Input: part model. Units: mm. Frame: model coordinates. A direction names the side the tool comes from. Coordinates: 2 decimals unless noted, no trailing zeros. Order: outer loops, then holes, each group sorted by start corner. A loop starts at its lowest first (then second) coordinate and runs counter-clockwise, first axis right, second up.
Autodesk Inventor part; units mm, degrees
ref_plane "YZ Plane" through (0, 0, 0) normal (1, 0, 0) x (0, 1, 0)
ref_plane "XZ Plane" through (0, 0, 0) normal (0, 1, 0) x (-1, 0, 0)
ref_plane "XY Plane" through (0, 0, 0) normal (0, 0, 1) x (1, 0, 0)
sketch "Boceto1" plane through (0, 0, 0) normal (0, 0, 1) x (1, 0, 0)
  line L0 (-19.271, 0) -> (-1.6402, 0)
  circle A0 centre (-16, 0) radius 2.75
  circle A1 centre (16, 0) radius 2.75
  line L1 (21, -7) -> (-21, -7)
  line L2 (-21, -7) -> (-21, 7)
  line L3 (-21, 7) -> (21, 7)
  line L4 (21, 7) -> (21, -7)
  line L5 (21, -7) -> (-21, 7) construction
  line L6 (-21, -7) -> (21, 7) construction
  point P0 (0, 0)
  point P1 (0, 0)
  dimension "d0" = 5.5
  dimension "d1" = 5.5
  dimension "d2" = 16
  dimension "d3" = 32
  dimension "d4" = 14
  dimension "d5" = 42
extrude "Extrusión1" add sketch "Boceto1" along normal blind 6
sketch "Boceto2" plane through (0, 0, 6) normal (0, 0, 1) x (1, 0, 0)
  point P0 (0, 0)
sketch "Boceto3" plane through (0, 0, 0) normal (0, 1, 0) x (-1, 0, 0)
  line L0 (-21, 0) -> (21, 0)
  line L1 (-8.586, 32.8) -> (-8.586, 0)
  line L2 (-8.586, 0) -> (9.414, 0)
  line L3 (9.414, 0) -> (9.414, 32.8)
  arc A0 (-0.25, 23.9922) -> (0.25, 23.9922) centre (0, 20) ccw
  line L4 (0.25, 36.8) -> (-0.25, 36.8)
  line L5 (-0.25, 32.8) -> (-0.25, 22.8)
  line L6 (-0.25, 22.8) -> (0.25, 22.8)
  line L7 (0.25, 22.8) -> (0.25, 32.8)
  line L8 (0.25, 36.8) -> (-0.25, 22.8) construction
  line L9 (-0.25, 36.8) -> (0.25, 22.8) construction
  line L10 (9.414, 32.8) -> (0.25, 32.8)
  line L11 (-0.25, 32.8) -> (-8.586, 32.8)
  point P0 (0, 0)
  dimension "d8" = 32.8
  dimension "d9" = 8
  dimension "d10" = 20
  dimension "d12" = 18
  dimension "d13" = 0.5
  dimension "d14" = 14
extrude "Extrusión2" add sketch "Boceto3" against normal mid plane 14 contours L1 L11 L5 A0 L7 L10 L3 L0
fillet "Empalme1" radius 0.3 20 edges at (-4.832, -7, 32.8) (4.418, -7, 32.8) (-15.207, -7, 6) (14.793, -7, 6) (-21, 0, 6) (-21, 7, 3) (-21, -7, 3) (21, -7, 3) (21, 7, 3) (14.793, 7, 6) (21, 0, 6) (-15.207, 7, 6) (8.586, 0, 32.8) (-9.414, 0, 32.8) (8.586, 7, 19.4) (-9.414, 7, 19.4) (8.586, -7, 19.4) (-9.414, -7, 19.4) (-4.832, 7, 32.8) (4.418, 7, 32.8)
sketch "Boceto5" plane through (0, 0, 0) normal (1, 0, 0) x (0, 1, 0)
  circle A0 centre (-0.6204, 28.4) radius 2.25
  line L0 (6.7, 0) -> (-6.7, 0)
  point P0 (0, 0)
  dimension "d18" = 4.5
  dimension "d19" = 28.4
extrude "Extrusión3" cut sketch "Boceto5" along normal mid plane 20
properties part number "SK8_LinearShaftSupport" material "Aluminum 6061"
Item 1: Pin query (flat end, axial travel): pin 1 Ø6.5 at (y, z) = (-2, 16) entering from +X; pin 2 Ø5 at (x, y) = (-16, 0) entering from -Z; pin 3 Ø5.5 at (x, y) = (-14, 0.5) entering from +Z; pin 4 Ø5 at (y, z) = (-4, 21) entering from -X. Return the tip coordinate at first contact, or that it passes through.
Response values:
pin 1: stops at x = 8.59
pin 2: passes through
pin 3: stops at z = 6
pin 4: stops at x = -9.41
Item 2: Cut plane A-A on z = 28.4. Return loops of the section in (x, y), then the cut area to 3 significant figures.
Response values:
outline: (-9.41, -6.7) arc R0.3 ccw to (-9.11, -7) - (-0.25, -7) - (-0.25, -2.87) - (-9.41, -2.87) - close; (-9.41, 1.63) - (-0.25, 1.63) - (-0.25, 7) - (-9.11, 7) arc R0.3 ccw to (-9.41, 6.7) - close; (0.25, -7) - (8.29, -7) arc R0.3 ccw to (8.59, -6.7) - (8.59, -2.87) - (0.25, -2.87) - close; (0.25, 1.63) - (8.59, 1.63) - (8.59, 6.7) arc R0.3 ccw to (8.29, 7) - (0.25, 7) - close
area: 166 mm2
Item 3: Cut plane D-D on z = 3.5. Return loops of the section in (x, y).
Response values:
outline: (-21, -6.7) arc R0.3 ccw to (-20.7, -7) - (20.7, -7) arc R0.3 ccw to (21, -6.7) - (21, 6.7) arc R0.3 ccw to (20.7, 7) - (-20.7, 7) arc R0.3 ccw to (-21, 6.7) - close; hole circle Ø5.5 at (-16, 0); hole circle Ø5.5 at (16, 0)
Item 4: Cut plane C-C on x = -4.5. Return loops of the section in (y, z), then the cut area to 3 significant figures.
Response values:
outline: (-7, 0) - (7, 0) - (7, 32.5) arc R0.3 ccw to (6.7, 32.8) - (-6.7, 32.8) arc R0.3 ccw to (-7, 32.5) - close; hole circle Ø4.5 at (-0.62, 28.4)
area: 443 mm2
Item 5: Cut plane B-B on y = 0.5. Count the separate pieces of the cut face and the enclosed holes in it, then the cut area to 3 significant figures.
Response values:
separate pieces: 5
enclosed holes: 0
area: 546 mm2
Item 6: Draft query along Y for faces 1 (the face through (0, -7, 12)), 2 (the face through (-5, 0, 32.8)), 3 (the face through (-4.8, -1.1, 26.2)). Return one class per face: pulls with the +Y half, pulls with the -Y half, needs draft (parallel to the pull), parting line crosses it, or undercut.
Response values:
face 1: pulls with the -Y half
face 2: needs draft
face 3: undercut
Item 7: Ray query, probe 1 along X at (y, z) = (-3, 31); probe 2 along Y at (x, z) = (16, 3); probe 3 along X at (y, z) = (-0.5, 20). Return the intervals inside material, ascending.
Response values:
probe 1: x = -9.41 to -0.25, 0.25 to 8.59
probe 2: y = -7 to -2.75, 2.75 to 7
probe 3: x = -9.41 to -4, 4 to 8.59
Item 8: Access query for faces 4 (the face through (0.25, 2, 28)), 5 (the face through (8.586, 0, 19)), 6 (the face through (-13, 0, 6)). Directions: +Z, -Z, +X, -X, +Y, -Y. A direction counts if a zero-diameter tool reaches every point of the face in a straight line with its end or side. Return the directions, or none.
Response values:
face 4: +Z, +Y, -Y
face 5: +Z, +X, +Y, -Y
face 6: +Z, -X, +Y, -Y
